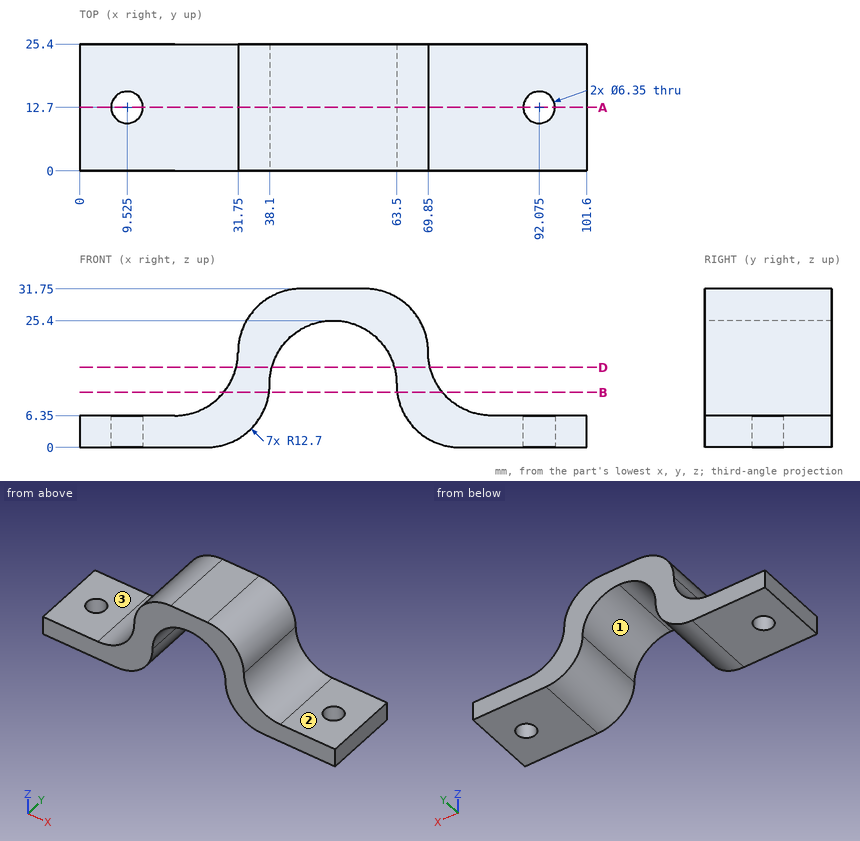
Check sheet for the drawn part. Datum: minimum x, y, z corner. Units: mm. A direction names the side the tool comes from. Coordinates: 2 decimals unless noted, no trailing zeros. Loops run counter-clockwise (first coordinate to the right, second up) from the corner with the lowest first, then second, coordinate; pieces in that order, holes last. Notation, with made-up numbers: (58, -14.75) -> (117, -14.75) arc R11 cw to (117, -0.75) -> close; hole circle Ø6 at (77, 78.5). An arc over 180 degrees is marked (long way). Answer in a Markdown table with one row per item.
1. Go/stop test with flat-tipped pins: pin 1 (2 mm diameter, centred on y = 11, z = 10.5, fed in from -X); pin 2 (12 mm diameter, centred on x = 69, y = 4.5, fed in from +Z); pin 3 (1.5 mm diameter, centred on y = 14.5, z = 24, fed in from -X); pin 4 (5 mm diameter, centred on x = 92.075, y = 12.7, fed in from -Z). Record where each tip stops, or that it passes through.
Check values:
| item | result |
|---|---|
| pin 1 | stops at x = 27.42 |
| pin 2 | stops at z = 30.32 |
| pin 3 | stops at x = 32.46 |
| pin 4 | passes through |
2. Material ranges on line 1 along X through (y, z) = (3.75, 13.5); line 2 along X through (y, z) = (16.75, 22); line 3 along Z through (x, y) = (13, 21.5), recorded low to high. Write a range as [from, to].
Check values:
| item | result |
|---|---|
| line 1 | x = [30.47, 38.13], [63.47, 71.13] |
| line 2 | x = [32.1, 42.15], [59.45, 69.5] |
| line 3 | z = [0, 6.35] |
3. Sectioned sample at A-A, the plane y = 12.7. Give the number of separate pieces and of enclosed holes in the cut face, then the cut area to 3 significant figures.
Check values:
| item | result |
|---|---|
| separate pieces | 3 |
| enclosed holes | 0 |
| area | 887 mm2 |
4. Sectioned sample at D-D, the plane z = 16. Record the boundary of the cut face in (x, y), then the cut area to 3 significant figures.
Check values:
| item | result |
|---|---|
| outline | (31.38, 0) -> (38.54, 0) -> (38.54, 25.4) -> (31.38, 25.4) -> close; (63.06, 0) -> (70.22, 0) -> (70.22, 25.4) -> (63.06, 25.4) -> close |
| area | 364 mm2 |
5. Sectioned sample at B-B, the plane z = 11. Record the boundary of the cut face in (x, y).
Check values:
| item | result |
|---|---|
| outline | (28.87, 0) -> (37.99, 0) -> (37.99, 25.4) -> (28.87, 25.4) -> close; (63.61, 0) -> (72.73, 0) -> (72.73, 25.4) -> (63.61, 25.4) -> close |
6. Access from +Z, -Z, +X, -X, +Y, -Y to the whole of each face (thin tool, end or side, straight path). Record for the marked faces 1, 2 and 3.
Check values:
| item | result |
|---|---|
| face 1 | -Z, +Y, -Y |
| face 2 | +Z, +X, +Y, -Y |
| face 3 | +Z, -X, +Y, -Y |
